Work out the finished part from the listing and answer in its coordinate system (mm). A direction names the side the tool comes from. Round coordinates to 2 decimals unless told otherwise and drop trailing zeros. Loops run counter-clockwise (first coordinate to the right, second up) from the corner with the lowest first, then second, coordinate; pieces in that order, holes last. Notation, with made-up numbers: (-14.5, -11.5) -> (-2.5, -11.5) arc R31 cw to (-2.5, 23.5) -> close; hole circle Ø9 at (-1, -15). An arc over 180 degrees is marked (long way). Use one line per item in the form item = value.
```python
from build123d import *

# Parameters (mm, degrees)
SKETCH1_W           = 25
SKETCH1_H           = 25
BOSS_EXTRUDE3_DEPTH = 25
SKETCH3_R           = 1.5
CUT_EXTRUDE1_DEPTH  = 7
SKETCH4_R           = 1.5
CUT_EXTRUDE2_DEPTH  = 7
SKETCH5_R           = 1.5
CUT_EXTRUDE3_DEPTH  = 7
CUT_EXTRUDE4_START  = -7
SKETCH6_R           = 1.5
CUT_EXTRUDE4_DEPTH  = 7
SKETCH7_R           = 1.5
CUT_EXTRUDE5_DEPTH  = 7


with BuildPart() as part:
    # Sketch1 → Boss-Extrude3 (new body)
    with BuildSketch(Plane.XY):
        Rectangle(SKETCH1_W, SKETCH1_H)
    extrude(amount=BOSS_EXTRUDE3_DEPTH)

    # Sketch3 → Cut-Extrude1 (cut)
    with BuildSketch(Plane(origin=(0, 12.5, 0), x_dir=(1, 0, 0), z_dir=(0, 1, 0))):
        with Locations(Location((0, -12.5, 0), (0, 0, 270))):
            Circle(SKETCH3_R)
    extrude(amount=-CUT_EXTRUDE1_DEPTH, mode=Mode.SUBTRACT)

    # Sketch4 → Cut-Extrude2 (cut)
    with BuildSketch(Plane.XY.offset(25)):
        Circle(SKETCH4_R)
    extrude(amount=-CUT_EXTRUDE2_DEPTH, mode=Mode.SUBTRACT)

    # Sketch5 → Cut-Extrude3 (cut)
    with BuildSketch(Plane(origin=(12.5, 0, 0), x_dir=(0, 0, -1), z_dir=(1, 0, 0))):
        with Locations((-12.656245037, 0)):
            Circle(SKETCH5_R)
    extrude(amount=-CUT_EXTRUDE3_DEPTH, mode=Mode.SUBTRACT)

    # Sketch6 → Cut-Extrude4 (cut)
    with BuildSketch(Plane(origin=(0, 0, 0), x_dir=(-1, 0, 0), z_dir=(0, 0, -1)).offset(CUT_EXTRUDE4_START)):
        with Locations(Location((0, 0, 0), (0, 0, 180))):
            Circle(SKETCH6_R)
    extrude(amount=CUT_EXTRUDE4_DEPTH, mode=Mode.SUBTRACT)

    # Sketch7 → Cut-Extrude5 (cut)
    with BuildSketch(Plane.ZY.offset(12.5)):
        with Locations((12.5, 0)):
            Circle(SKETCH7_R)
    extrude(amount=-CUT_EXTRUDE5_DEPTH, mode=Mode.SUBTRACT)


solid = part.part
```
(1) For faces 5 (the flat face through (0, 0, 7)), 6 (the cylindrical face through (0, 9, 11)), 7 (the flat face through (-5.5, 0, 12)), determine the directions among +Z, -Z, +X, -X, +Y, -Y from which every point of the face is accessible in a straight line to the end or side of a thin tool.
Completed:
face_5 = -Z
face_6 = +Y
face_7 = -X
(2) Find section A-A, the plane x = 0. Write down the section's boundary in (y, z), then the cut area to 3 significant figures.
Completed:
outline = (-12.5, 0) -> (-1.5, 0) -> (-1.5, 7) -> (1.5, 7) -> (1.5, 0) -> (12.5, 0) -> (12.5, 11) -> (5.5, 11) -> (5.5, 14) -> (12.5, 14) -> (12.5, 25) -> (1.5, 25) -> (1.5, 18) -> (-1.5, 18) -> (-1.5, 25) -> (-12.5, 25) -> close
area = 562 mm2
(3) Consider L1, parallel to Y at x = 0, z = 22.75; L2, parallel to Z at x = 5.75, y = 0.25. Determine where each line is inside the solid, lowest interval first.
Completed:
L1 = -12.5 to -1.5, 1.5 to 12.5
L2 = 0 to 11.18, 14.14 to 25
(4) Find section C-C, the plane z = 12.5. Write down the section's boundary in (x, y), then the cut area to 3 significant figures.
Completed:
outline = (-12.5, -12.5) -> (12.5, -12.5) -> (12.5, -1.49) -> (5.5, -1.49) -> (5.5, 1.49) -> (12.5, 1.49) -> (12.5, 12.5) -> (1.5, 12.5) -> (1.5, 5.5) -> (-1.5, 5.5) -> (-1.5, 12.5) -> (-12.5, 12.5) -> (-12.5, 1.5) -> (-5.5, 1.5) -> (-5.5, -1.5) -> (-12.5, -1.5) -> close
area = 562 mm2
(5) Find section B-B, the plane y = 0. Write down the section's boundary in (x, z).
Completed:
outline = (-12.5, 0) -> (-1.5, 0) -> (-1.5, 7) -> (1.5, 7) -> (1.5, 0) -> (12.5, 0) -> (12.5, 11.16) -> (5.5, 11.16) -> (5.5, 14.16) -> (12.5, 14.16) -> (12.5, 25) -> (1.5, 25) -> (1.5, 18) -> (-1.5, 18) -> (-1.5, 25) -> (-12.5, 25) -> (-12.5, 14) -> (-5.5, 14) -> (-5.5, 11) -> (-12.5, 11) -> close
(6) For a pull along Z with two mould halves and no side action, classify faces 1 (the cylindrical face through (9.05, -0.57, 11.27)), 2 (the flat face through (5.5, 0, 13)), 3 (the flat face through (0, -12.5, 12)), 4 (the flat face through (0, 3, 25)) as +Z half, -Z half, draft (parallel to the pull), parting line (faces both ways), or undercut.
Completed:
face_1 = undercut
face_2 = undercut
face_3 = draft
face_4 = +Z half
(7) Given P1, Ø2.5, axis at x = 0, y = 0, coming from the -Z side; P2, Ø2.5, axis at x = 0, y = 0, coming from the +Z side, each flat-ended and moving along its own axis, determine where each tip first touches the part or whether it passes through.
Completed:
P1 = 7
P2 = 18
